Verification items for this drawing (mm, ordinates from the low corner). Coordinates: 2 decimals unless noted, no trailing zeros. Order: outer loops, then holes, each group sorted by start corner. A loop starts at its lowest first (then second) coordinate and runs counter-clockwise, first axis right, second up. Notation, with made-up numbers: (-17, 1.5) -> (26, 1.5) arc R27 ccw to (26, 25.5) -> close; hole circle Ø10 at (-18, 80). An arc over 180 degrees is marked (long way). Answer as CSV lines item,"result". Start each with the question number.
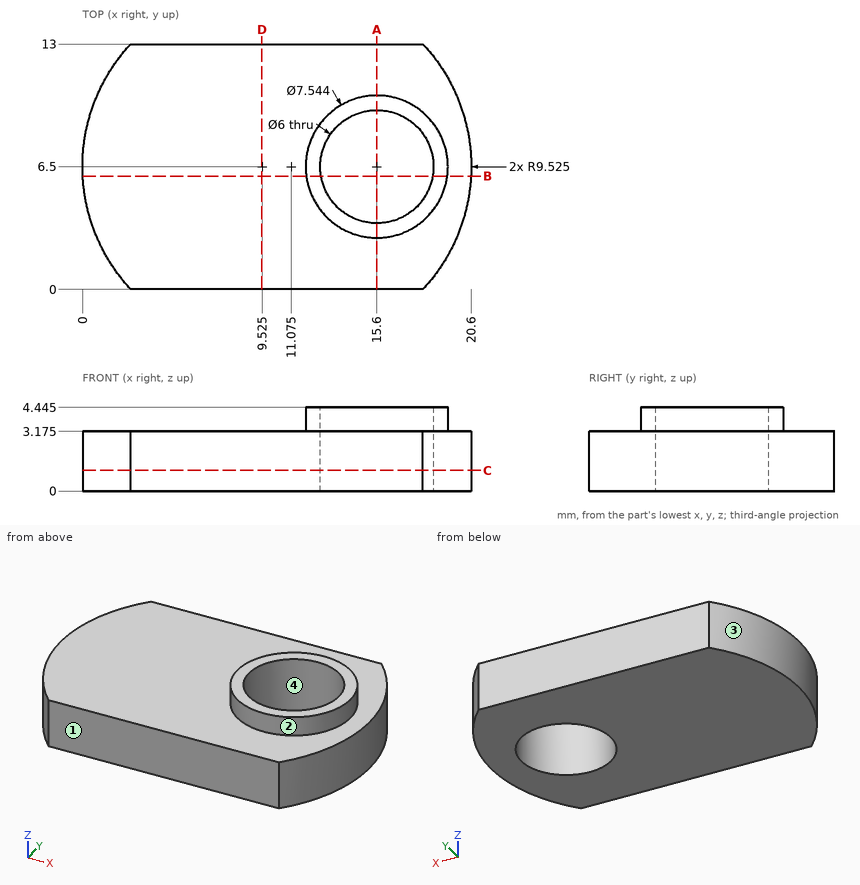
Q1. Go/stop test with flat-tipped pins: pin 1 Ø6.5 at (x, y) = (10.5, 7.5) entering from +Z (3 decimals); pin 2 Ø1.5 at (y, z) = (4.5, 1) entering from -X; pin 3 Ø5 at (x, y) = (15.6, 6.5) entering from +Z. Record where each tip stops, or that it passes through.
Q2. Release check for a two-part mould opening along X. For the marked faces 1, 2, 3 and 4 record: released by +X, released by -X, zero draft, split by the parting line, or undercut.
Q3. Sectioned sample at B-B, the plane y = 6. Record the cut outline in (x, z) (3 decimals), then the cut area to 3 significant figures.
Q4. Sectioned sample at A-A, the plane x = 15.6. Record the cut outline in (y, z) (3 decimals).
Q5. Sectioned sample at D-D, the plane x = 9.5. Record the cut outline in (y, z) (3 decimals), then the cut area to 3 significant figures.
Q6. Sectioned sample at C-C, the plane z = 1.1. Record the cut outline in (x, y) (3 decimals), then the cut area to 3 significant figures.
Q7. Thickness scan on L1, parallel to Y at x = 15.6, z = 1.5; L2, parallel to Z at x = 12, y = 4 (3 decimals); L3, parallel to Y at x = 17.5, z = 2. Record the ranges inside material, lowest first.
Geometry results:
1,pin 1,"stops at z = 4.445"
1,pin 2,"stops at x = 0.08"
1,pin 3,"passes through"
2,face 1,"zero draft"
2,face 2,"split by the parting line"
2,face 3,"released by -X"
2,face 4,"undercut"
3,outline,"(0.013, 0) -> (12.642, 0) -> (12.642, 4.445) -> (11.861, 4.445) -> (11.861, 3.175) -> (0.013, 3.175) -> close; (18.558, 0) -> (20.587, 0) -> (20.587, 3.175) -> (19.339, 3.175) -> (19.339, 4.445) -> (18.558, 4.445) -> close"
3,area,"48.5 mm^2"
4,outline,"(0, 0) -> (3.5, 0) -> (3.5, 4.445) -> (2.728, 4.445) -> (2.728, 3.175) -> (0, 3.175) -> close; (9.5, 0) -> (13, 0) -> (13, 3.175) -> (10.272, 3.175) -> (10.272, 4.445) -> (9.5, 4.445) -> close"
5,outline,"(0, 0) -> (13, 0) -> (13, 3.175) -> (0, 3.175) -> close"
5,area,"41.3 mm^2"
6,outline,"(2.563, 0) -> (18.037, 0) arc R9.525 ccw to (18.037, 13) -> (2.563, 13) arc R9.525 ccw to start; hole circle Ø6 at (15.6, 6.5)"
6,area,"219 mm^2"
7,L1,"y = 0 to 3.5, 9.5 to 13"
7,L2,"z = 0 to 3.175"
7,L3,"y = 0 to 4.18, 8.82 to 13"
